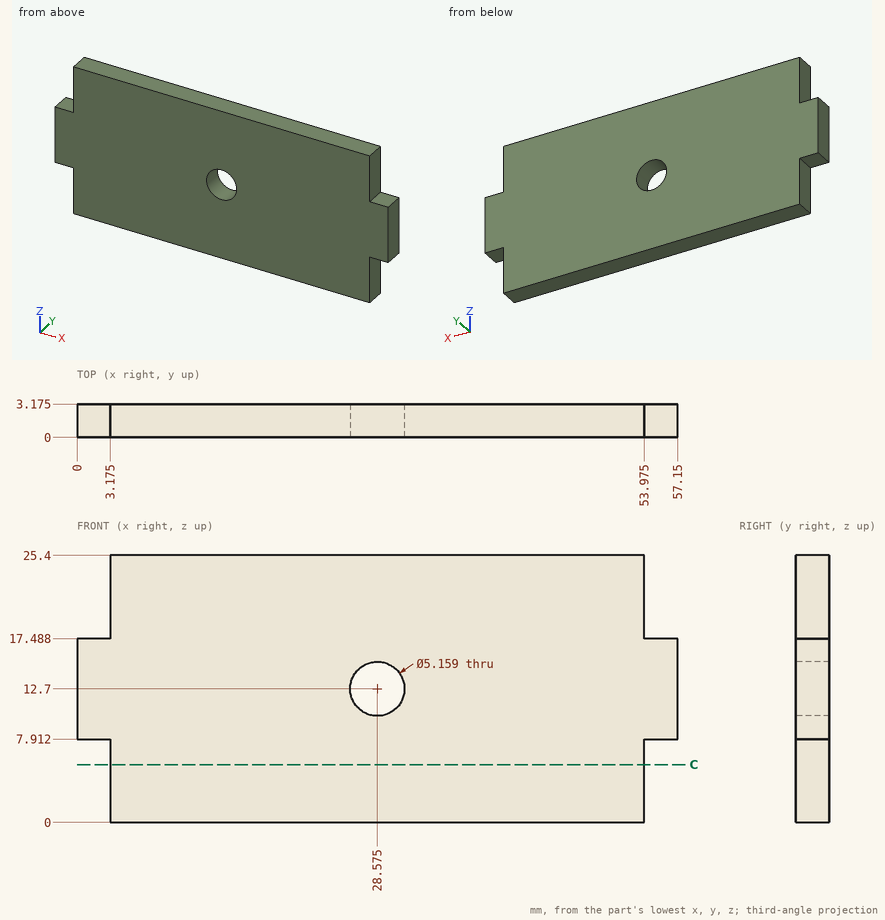
Geometry check sheet. Reference: drawing and pictorial views, mm from the part's lowest x, y, z. Give positions to 0.01 mm unless a question says otherwise; leave off trailing zeros. Loops run counter-clockwise (first coordinate to the right, second up) from the corner with the lowest first, then second, coordinate; pieces in that order, holes last. Notation, with made-up numbers: M 88,79 L 105,79 A8 cw 105,85 Z; hole C -19.75,-33.75 d6. An arc over 180 degrees is marked long. Use a Markdown table: item, result. Add a question column.
Q1. Sectioned sample at C-C, the plane z = 5.5. Record the cut outline in (x, y) (1 decimal).
Q2. Scan lines: line 1 along Z through (x, y) = (28, 3) (1 decimal); line 2 along X through (y, z) = (2.15, 22) (1 decimal); line 3 along Z through (x, y) = (30.5, 0.3) (1 decimal). Record each from-to range of solid material in increasing order. Write a range as [from, to].
Q3. Go/stop test with flat-tipped pins: pin 1 (1 mm diameter, centred on x = 1, y = 1, fed in from -Z); pin 2 (1 mm diameter, centred on y = 2, z = 3, fed in from +X) (3 decimals); pin 3 (1.5 mm diameter, centred on x = 19.5, y = 1, fed in from -Z); pin 4 (1.6 mm diameter, centred on y = 2, z = 5.5, fed in from -X) (3 decimals). Record where each tip stops, or that it passes through.
Verdict:
| question | item | result |
|---|---|---|
| 1 | outline | M 3.2,0 L 54,0 L 54,3.2 L 3.2,3.2 Z |
| 2 | line 1 | [0, 10.2], [15.2, 25.4] |
| 2 | line 2 | [3.2, 54] |
| 2 | line 3 | [0, 11], [14.4, 25.4] |
| 3 | pin 1 | z = 7.91 |
| 3 | pin 2 | x = 53.975 |
| 3 | pin 3 | z = 0 |
| 3 | pin 4 | x = 3.175 |
